from build123d import *

# Parameters (mm, degrees)
SKETCH1_R           = 11
BOSS_EXTRUDE1_DEPTH = 10
SKETCH2_R           = 20
BOSS_EXTRUDE2_DEPTH = 45
CUT_EXTRUDE1_DEPTH  = 54.150729064
SKETCH5_R           = 7.125
CUT_EXTRUDE2_DEPTH  = 54.150729224
CUT_EXTRUDE3_START  = -45
CUT_EXTRUDE3_DEPTH  = 45


with BuildPart() as part:
    # Sketch1 → Boss-Extrude1 (new body)
    with BuildSketch(Plane.XY):
        Circle(SKETCH1_R)
    extrude(amount=BOSS_EXTRUDE1_DEPTH)

    # Sketch2 → Boss-Extrude2 (add)
    with BuildSketch(Plane(origin=(0, 0, 0), x_dir=(-1, 0, 0), z_dir=(0, 0, -1))):
        with Locations(Location((0, 0, 0), (0, 0, 180))):
            Circle(SKETCH2_R)
    extrude(amount=BOSS_EXTRUDE2_DEPTH)

    # Sketch3 → Cut-Extrude1 (cut, through all)
    with BuildSketch(Plane(origin=(0, 0, 0), x_dir=(0, 0, -1), z_dir=(1, 0, 0))):
        with BuildLine():
            Line((75.441676997, 14.75), (25.441676997, 14.75))
            ThreePointArc((25.441676997, 14.75), (10.816676997, 0.125), (25.441676997, -14.5))
            Line((25.441676997, -14.5), (75.441676997, -14.5))
            Line((75.441676997, -14.5), (75.441676997, 14.75))
        make_face()
    extrude(amount=-CUT_EXTRUDE1_DEPTH, mode=Mode.SUBTRACT)

    # Sketch5 → Cut-Extrude2 (cut, through all)
    with BuildSketch(Plane.ZY):
        with Locations((-25.816676997, 0.125)):
            Circle(SKETCH5_R)
    extrude(amount=-CUT_EXTRUDE2_DEPTH, mode=Mode.SUBTRACT)

    # Sketch6 → Cut-Extrude3 (cut)
    with BuildSketch(Plane(origin=(0, 0, -45), x_dir=(-1, 0, 0), z_dir=(0, 0, -1)).offset(CUT_EXTRUDE3_START)):
        with BuildLine():
            Line((-11.346386998, 16.469957562), (-11.346386998, -16.469957562))
            ThreePointArc((-11.346386998, -16.469957562), (-20, 0), (-11.346386998, 16.469957562))
        make_face()
    extrude(amount=CUT_EXTRUDE3_DEPTH, mode=Mode.SUBTRACT)


solid = part.part
Geometry check sheet. Reference: the model listing, model coordinates, mm. A direction names the side the tool comes from. Give positions to 0.01 mm unless a question says otherwise; leave off trailing zeros. Write each loop counter-clockwise with the first axis right and the second up, starting at its lowest first coordinate (ties: lowest second). Pieces come first, ordered by that corner, then holes. Notation, with made-up numbers: M -20,-29 L 0,-29 A19 cw 0,3 Z; hole C 12,53.5 d2. An arc over 180 degrees is marked long. Answer as CSV lines item,"result". Start each with the question number.
Q1. Section check D-D, the plane z = 4. Record the cut outline in (x, y).
Q2. Section check B-B, the plane z = -19.5. Record the cut outline in (x, y).
Q3. Section check A-A, the plane y = 3. Record the cut outline in (x, z), then the cut area to 3 significant figures.
Q4. Go/stop test with flat-tipped pins: pin 1 (5 mm diameter, centred on y = -7, z = -22.5, fed in from -X); pin 2 (12 mm diameter, centred on x = -10.5, z = -8.5, fed in from +Y); pin 3 (2 mm diameter, centred on x = -8.5, y = 6.5, fed in from -Z). Record where each tip stops, or that it passes through.
Q5. Release check for a two-part mould opening along Y. For faces 1 (the face through (-10.862, -16.793, -22.185)), 2 (the face through (-7, -14.5, -35)), 3 (the face through (4, 0, -45)), 4 (the face through (-7.64, 0.45, -10.82)) record: pulls with the +Y half, pulls with the -Y half, needs draft (parallel to the pull), parting line crosses it, or undercut.
Q6. Material ranges on L1, parallel to Z at x = 8, y = 0.5; L2, parallel to Y at x = -9.5, z = -22; L3, parallel to Y at x = -7.5, z = -14.5, recorded low to high.
Q7. Tool access check on faces 5 (the face through (-2.38, -10.74, 4.93)), 6 (the face through (5.594, 2.265, -19.021)), 7 (the face through (-7, 14.75, -35)). Record the directions out of +Z, -Z, +X, -X, +Y, -Y that give a thin tool (end or side, any length) a straight path to the whole face; none if there is none.
Q8. Section check C-C, the plane x = -5.5. Record the cut outline in (y, z) (3 decimals), then the cut area to 3 significant figures.
Geometry says:
1,outline,"C 0,0 d22"
2,outline,"M -14.99,-13.24 A20 ccw 11.35,-16.47 L 11.35,-3.17 L 0,-3.17 L 0,-13.24 Z; M -14.77,13.49 L 0,13.49 L 0,3.42 L 11.35,3.42 L 11.35,16.47 A20 ccw Z"
3,outline,"M -19.77,-11.1 L 0,-11.1 L 0,-19.3 L 11.35,-19.3 L 11.35,0 L 10.58,0 L 10.58,10 L -10.58,10 L -10.58,0 L -19.77,0 Z; M 0,-45 L 11.35,-45 L 11.35,-32.34 L 0,-32.34 Z"
3,area,"794 mm^2"
4,pin 1,"x = 0"
4,pin 2,"y = 19.49"
4,pin 3,"z = -12.81"
5,face 1,"parting line crosses it"
5,face 2,"undercut"
5,face 3,"needs draft"
5,face 4,"undercut"
6,L1,"-45 to -32.93, -18.7 to 10"
6,L2,"-17.6 to -14.09, 14.34 to 17.6"
6,L3,"-18.54 to -9.58, 9.83 to 18.54"
7,face 5,"+Z"
7,face 6,"+X, -X"
7,face 7,"-Z, -X"
8,outline,"M -19.229,-45 L -14.5,-45 L -14.5,-25.442 A14.625 cw 14.75,-25.442 L 14.75,-45 L 19.229,-45 L 19.229,0 L 9.526,0 L 9.526,10 L -9.526,10 L -9.526,0 L -19.229,0 Z"
8,area,"1,010 mm^2"
